```python
from build123d import *

# Parameters (mm, degrees)
SKETCH2_W           = 150
SKETCH2_H           = 60
EXTRUDE1_DEPTH      = 20
SKETCH3_W           = 20.4
SKETCH3_H           = 20.4
EXTRUDE2_DEPTH      = 20
EXTRUDE3_DEPTH      = 10
EXTRUDE4_DEPTH      = 98.418669917
EXTRUDE4_DEPTH_BACK = 98.418669917
SKETCH5_W           = 75
SKETCH5_H           = 27.596189432
SKETCH6_W           = 20
SKETCH6_H           = 20
EXTRUDE5_DEPTH      = 20
FILLET1_R           = 2


with BuildPart() as part:
    # Sketch2 → Extrude1 (new body)
    with BuildSketch(Plane(origin=(0, 0, 0), x_dir=(1, 0, 0), z_dir=(0, 1, 0))):
        Rectangle(SKETCH2_W, SKETCH2_H)
    extrude(amount=EXTRUDE1_DEPTH)

    # Sketch3 → Extrude2 (cut)
    with BuildSketch(Plane(origin=(0, 20, 0), x_dir=(1, 0, 0), z_dir=(0, 1, 0))):
        with Locations((0, 12.9)):
            Rectangle(SKETCH3_W, SKETCH3_H)
        with Locations((0, -12.9)):
            Rectangle(SKETCH3_W, SKETCH3_H)
    extrude(amount=-EXTRUDE2_DEPTH, mode=Mode.SUBTRACT)

    # Sketch4 → Extrude3 (add, symmetric)
    with BuildSketch(Plane.XY):
        Polygon((-75, 20), (-75, 47.596189432), (-40, 38.217967697), (-40, 20), align=None)
    extrude3 = extrude(amount=EXTRUDE3_DEPTH, both=True)

    # Mirror1: Extrude3 across plane
    add(extrude3.mirror(Plane(origin=(0, 0, 0), x_dir=(0, 0, 1), z_dir=(1, 0, 0))))

    # Sketch5 → Extrude4 (cut, two sides: drawn at the far end of the back side and taken through both)
    with BuildSketch(Plane(origin=(0, 0, -10), x_dir=(-1, 0, 0), z_dir=(0, 0, -1)).offset(-EXTRUDE4_DEPTH_BACK)):
        Polygon((-40, 20), (-75, 20), (-75, 0), (75, 0), (75, 20), (0, 20), align=None)
        with Locations((37.5, 33.798094716)):
            Rectangle(SKETCH5_W, SKETCH5_H)
    extrude(amount=EXTRUDE4_DEPTH + EXTRUDE4_DEPTH_BACK, mode=Mode.SUBTRACT)

    # Sketch6 → Extrude5 (add)
    with BuildSketch(Plane.XZ.offset(-20)):
        with Locations((57.5, 0)):
            Rectangle(SKETCH6_W, SKETCH6_H)
    extrude(amount=EXTRUDE5_DEPTH)

    # Fillet1
    fillet1_edges = [part.edges().sort_by_distance(p)[0] for p in [
        (75, 47.596189432, 0),
        (40, 38.217967697, 0),
    ]]
    fillet(fillet1_edges, radius=FILLET1_R)


solid = part.part
```
Here's how the part is built. I have some questions about the finished solid (model axes, mm). A direction names the side the tool comes from. Give positions to 0.01 mm unless a question says otherwise; leave off trailing zeros. Loops run counter-clockwise (first coordinate to the right, second up) from the corner with the lowest first, then second, coordinate; pieces in that order, holes last. Notation, with made-up numbers: M 83,-24.75 L 117,-24.75 A20 ccw 117,0.25 Z; hole C 32,-39 d5. An arc over 180 degrees is marked long. Use one line per item in the form item = value. Start each with the question number.
Q1. Which directions (+Z, -Z, +X, -X, +Y, -Y) give clear straight access to the entire face, cutting with the end or side of a thin tool? Please do faces 1 (the flat face through (67.5, 10, 0)), 2 (the flat face through (44, 20, 0)), 3 (the flat face through (57, 0, 0)).
Q2. If we section it at A-A (z = 0.25): Write out the boundary of the cut face in (x, y), then the cut area to 3 significant figures.
Q3. If we section it at B-B (y = 13.5): Write out the boundary of the cut face in (x, z), then the cut area to 3 significant figures.
Q4. If we section it at C-C (x = 45): Write out the boundary of the cut face in (y, z), then the cut area to 3 significant figures.
Q5. I need wall thicknesses on line 1 along X through (y, z) = (3.5, -9); line 2 along Y through (x, z) = (63, -3.75); line 3 along Y through (x, z) = (52.5, 6). Which ranges of each line are inside material? Lowest first, please.
Q6. Will these pins go through, and if not, where does the flat tip stop? pin 1 Ø2 at (x, z) = (43, 1.5) entering from -Y; pin 2 Ø6 at (x, z) = (63, -2.5) entering from -Y; pin 3 Ø1.5 at (y, z) = (13, 7.5) entering from -X; pin 4 Ø3 at (y, z) = (13.5, 0.5) entering from +X.
Taken from the geometry:
q1.face_1 = +Z, -Z, +X, -Y
q1.face_2 = +Z, -Z, -X, -Y
q1.face_3 = +Z, -Z, +X, -X, -Y
q2.outline = M 40,20 L 47.5,20 L 47.5,0 L 67.5,0 L 67.5,20 L 75,20 L 75,44.99 A2 ccw 72.48,46.92 L 41.48,38.62 A2 ccw 40,36.68 Z
q2.area = 1,200 mm^2
q3.outline = M 47.5,-10 L 67.5,-10 L 67.5,10 L 47.5,10 Z
q3.area = 400 mm^2
q4.outline = M 20,-10 L 39.56,-10 L 39.56,10 L 20,10 Z
q4.area = 391 mm^2
q5.line_1 = 47.5 to 67.5
q5.line_2 = 0 to 44.38
q5.line_3 = 0 to 41.57
q6.pin_1 = 20
q6.pin_2 = 0
q6.pin_3 = 47.5
q6.pin_4 = 67.5
